Input: part model. Units: mm. Frame: model coordinates. A direction names the side the tool comes from. Round coordinates to 2 decimals unless told otherwise and drop trailing zeros. Order: outer loops, then holes, each group sorted by start corner. A loop starts at its lowest first (then second) coordinate and runs counter-clockwise, first axis right, second up.
Item 1: Mould query, pull axis X, two halves, no side actions, for faces 4 (the flat face through (-10.134, 25, 12)), 5 (the flat face through (5, 28, 25.733)), 6 (the flat face through (17, 19.7, 15)). Classes: released by +X, released by -X, zero draft, split by the parting line, or undercut.
Item 2: Cut plane B-B on x = -0.5. Output: boundary loops of the cut face in (y, z).
Item 3: Reachability of faces 1 (the flat face through (5, 21, 6)), 2 (the flat face through (5.08, 26.44, 26.49)), 3 (the flat face through (5, 28, -1.733)) from +Z, -Z, +X, -X, +Y, -Y: full face, straight path, thin tool, end or side. Return the list, or none.
Item 4: First-contact query: pin 1 (1.5 mm diameter, centred on x = 9.5, z = 4.5, fed in from -Y); pin 2 (1 mm diameter, centred on x = 13, z = 3.5, fed in from +Y); pin 3 (3 mm diameter, centred on x = 15, y = 21, fed in from +Z). Flat tips, straight axial feed; report the tip coordinate or a pass-through.
Item 5: Cut plane A-A on z = 9.5. Output: boundary loops of the cut face in (x, y).
Item 6: Cut plane C-C on z = 20.5. Output: boundary loops of the cut face in (x, y).
Item 7: Line query: L1, parallel to Z at x = 6.5, y = 23; L2, parallel to X at y = 21.2, z = 17.3; L3, parallel to Y at x = 1, z = 17. Output: solid intervals per line, ascending.
Autodesk Inventor part; units mm, degrees
ref_plane "Work Plane3" through (-25.1344, 22.2348, 12) normal (0, 0, -1) x (1, 0, 0)
ref_plane "YZ Plane" through (0, 0, 0) normal (1, 0, 0) x (0, 1, 0)
ref_plane "XZ Plane" through (0, 0, 0) normal (0, 1, 0) x (-1, 0, 0)
sketch "Sketch1" plane through (0, 0, 0) normal (0, 0, 1) x (1, 0, 0)
  circle A0 centre (23.8656, 17.2) radius 3
  line L0 (34.8656, 12.9938) -> (34.8656, 22.2)
  line L1 (165.9417, 25.2) -> (-24.8583, 25.2)
  line L2 (34.8656, 25.2) -> (-24.8606, 25.2)
  line L3 (-24.8606, 25.2) -> (-24.8606, 10.2)
  line L4 (-24.8606, 10.2) -> (34.8656, 10.2)
  line L5 (34.8656, 10.2) -> (34.8656, 25.2)
  point P0 (0, 0)
  dimension "d0" = 15
extrude "Extrusion1" add sketch "Sketch1" along normal blind 4
sketch "Sketch2" plane through (0, 0, 4) normal (0, 0, 1) x (1, 0, 0)
  circle A0 centre (23.8656, 17.2) radius 3
  line L0 (17.8656, 17.2) -> (20.8656, 22.3962)
  line L1 (20.8656, 22.3962) -> (26.8656, 22.3962)
  line L2 (26.8656, 22.3962) -> (29.8656, 17.2)
  line L3 (29.8656, 17.2) -> (26.8656, 12.0038)
  line L4 (26.8656, 12.0038) -> (20.8656, 12.0038)
  line L5 (20.8656, 12.0038) -> (17.8656, 17.2)
  circle A1 centre (23.8656, 17.2) radius 3
  line L6 (34.8656, 25.2) -> (-24.8606, 25.2)
  line L7 (-24.8606, 25.2) -> (-24.8606, 10.2)
  line L8 (-24.8606, 10.2) -> (34.8656, 10.2)
  line L9 (34.8656, 10.2) -> (34.8656, 25.2)
  point P0 (0, 0)
extrude "Extrusion2" add sketch "Sketch2" along normal blind 4 contours L9 L8 L7 L6
sketch "Sketch4" plane through (34.8656, 10.2, 8) normal (1, 0, 0) x (0, 0, -1)
  line L0 (8, 0.0155) -> (-4, 0.0155)
  point P0 (8, -10.2)
  dimension "d8" = 12
sketch "Sketch6" plane through (0, 0, 4) normal (0, 0, 1) x (1, 0, 0)
  line L0 (20.8656, 22.3962) -> (17.8656, 17.2)
  line L1 (17.8656, 17.2) -> (20.8656, 12.0038)
  line L2 (20.8656, 12.0038) -> (26.8656, 12.0038)
  line L3 (26.8656, 12.0038) -> (29.8656, 17.2)
  line L4 (29.8656, 17.2) -> (26.8656, 22.3962)
  circle A0 centre (23.8656, 17.2) radius 3
  line L5 (26.8656, 22.3962) -> (20.8656, 22.3962)
  point P0 (0, 0)
extrude "Extrusion4" cut sketch "Sketch6" along normal blind 16
sketch "Sketch7" plane through (0, 0, 4) normal (0, 0, 1) x (1, 0, 0)
  circle A0 centre (23.8656, 17.2) radius 3
  line L0 (17.8656, 17.2) -> (20.8656, 12.0038)
  line L1 (17.8656, 17.2) -> (20.8656, 22.3962)
  line L2 (20.8656, 22.3962) -> (26.8656, 22.3962)
  line L3 (26.8656, 22.3962) -> (29.8656, 17.2)
  line L4 (29.8656, 17.2) -> (26.8656, 12.0038)
  line L5 (26.8656, 12.0038) -> (20.8656, 12.0038)
  line L6 (20.8656, 12.0038) -> (17.8656, 17.2)
  point P0 (0, 0)
extrude "Extrusion5" cut sketch "Sketch7" along normal blind 16
sketch "Sketch8" plane through (34.8656, 10.2, 0) normal (1, 0, 0) x (0, 0, -1)
  line L0 (-41.5, 15) -> (17.4652, 15)
  line L1 (17.4652, 16) -> (17.4652, 15) construction
  line L2 (15.4652, 18) -> (17.4652, 16) construction
  line L3 (14.5, 18) -> (15.4652, 18) construction
  line L4 (14.5, 18) -> (14.5, 63) construction
  arc A0 (14.5, 63) -> (12.5, 65) centre (12.5, 63) ccw construction
  line L5 (12.5, 65) -> (7.5, 65) construction
  line L6 (7.5, 65) -> (10.5, 62) construction
  line L7 (10.5, 62) -> (10.5, 20) construction
  arc A1 (8.5, 18) -> (10.5, 20) centre (8.5, 20) ccw construction
  line L8 (8.5, 18) -> (-32.5, 18) construction
  arc A2 (-34.5, 20) -> (-32.5, 18) centre (-32.5, 20) ccw construction
  line L9 (-34.5, 20) -> (-34.5, 62) construction
  line L10 (-34.5, 62) -> (-31.5, 65) construction
  line L11 (-31.5, 65) -> (-36.5, 65) construction
  arc A3 (-36.5, 65) -> (-38.5, 63) centre (-36.5, 63) ccw construction
  line L12 (-38.5, 63) -> (-38.5, 18) construction
  line L13 (-38.5, 18) -> (-39.5, 18) construction
  line L14 (-39.5, 18) -> (-41.5, 16) construction
  line L15 (-41.5, 16) -> (-41.5, 15) construction
  line L16 (0, 15) -> (17.4652, 15)
  line L17 (17.4652, 15) -> (18.4652, 15)
  line L18 (18.4652, 15) -> (18.4652, 16)
  line L19 (18.4652, 16) -> (15.4652, 19)
  line L20 (21.4652, 15) -> (21.4652, 18)
  line L21 (17.4652, 22) -> (15.4652, 22)
  line L22 (21.4652, 15) -> (21.4652, 12.0348)
  line L23 (21.4652, 12.0348) -> (0, 12.0348)
  line L24 (21.4652, 18) -> (17.4652, 22)
  line L25 (0, 0) -> (0, 15) construction
  line L26 (-32.6881, 12) -> (-32.6881, -32.4)
  line L27 (0, 12.0348) -> (-12, 12.0348)
  line L28 (-12, 15) -> (0, 15)
  arc A4 (-34.5, 20) -> (-32.5, 18) centre (-32.5, 20) ccw construction
  line L29 (-24, 15) -> (-41.4652, 15)
  line L30 (-41.4652, 15) -> (-42.4652, 15)
  line L31 (-42.4652, 15) -> (-42.4652, 16)
  line L32 (-42.4652, 16) -> (-39.4652, 19)
  line L33 (-45.4652, 15) -> (-45.4652, 18)
  line L34 (-41.4652, 22) -> (-39.4652, 22)
  line L35 (-45.4652, 15) -> (-45.4652, 12.0348)
  line L36 (-45.4652, 12.0348) -> (-24, 12.0348)
  line L37 (-45.4652, 18) -> (-41.4652, 22)
  line L38 (-24, 12.0348) -> (-12, 12.0348)
  line L39 (-12, 15) -> (-24, 15)
  line L40 (18.4652, 15) -> (-42.4652, 15)
  line L41 (21.4652, 12.0348) -> (-45.4652, 12.0348)
  line L42 (-45.4652, 12.0348) -> (-45.4652, 18)
  line L43 (-45.4652, 18) -> (-41.4652, 22)
  line L44 (-41.4652, 22) -> (-39.4652, 22)
  line L45 (-39.4652, 19) -> (-42.4652, 16)
  line L46 (-42.4652, 16) -> (-42.4652, 15)
  line L47 (-42.4652, 15) -> (18.4652, 15)
  line L48 (15.4652, 19) -> (15.4652, 22)
  line L49 (-39.4652, 19) -> (-39.4652, 22)
  point P0 (0, -10.2)
  point P1 (21.4652, 22)
  point P2 (-45.4652, 22)
  dimension "d16" = 3
  dimension "d17" = 4
  dimension "d18" = 4
extrude "Extrusion6" add sketch "Sketch8" against normal blind 60
sketch "Sketch9" plane through (34.8656, 22.2348, 8) normal (0, -1, 0) x (1, 0, 0)
  line L0 (0, -8) -> (0, -29.4652)
  line L1 (-60, -29.4652) -> (-60, 37.4652)
  line L2 (0, -8) -> (-60, -8)
  line L3 (-60, -8) -> (-60, 16)
  line L4 (-60, 16) -> (0, 16)
  line L5 (0, 16) -> (0, -8)
  line L6 (-60, 4) -> (0, 4)
  point P0 (-34.8656, -8)
  dimension "d21" = 24
ref_plane "Work Plane3" through (-25.1344, 22.2348, 12) normal (0, 0, -1) x (1, 0, 0)
mirror "Mirror2" about plane through (-25.1344, 22.2348, 12) normal (0, 0, -1) of "Extrusion1", "Extrusion2"
sketch "Sketch11" plane through (26.9587, 22.2348, 20) normal (0, 0, -1) x (-1, 0, 0)
  circle A0 centre (3.0931, -5.0348) radius 3
  circle A1 centre (3.0931, -5.0348) radius 7
  circle A2 centre (3.0931, -5.0348) radius 3
  line L0 (-3.9069, -5.0348) -> (-0.4069, 1.0273)
  line L1 (-0.4069, 1.0273) -> (6.5931, 1.0273)
  line L2 (6.5931, 1.0273) -> (10.0931, -5.0348)
  line L3 (10.0931, -5.0348) -> (6.5931, -11.097)
  line L4 (6.5931, -11.097) -> (-0.4069, -11.097)
  line L5 (-0.4069, -11.097) -> (-3.9069, -5.0348)
  point P0 (26.9587, -22.2348)
  dimension "d25" = 14
extrude "Extrusion8" cut sketch "Sketch11" along normal blind 16 contours L3 L4 L5 L0 L1 L2
scale "Scale1" factors (0.5, 0.5, 0.5) then translate (2.4328, 12.6, 6) bodies 1
properties part number "TopToBatteryJoint"
From the geometry:
1. face 4: released by -X
1. face 5: zero draft
1. face 6: undercut
2. outline: (17.7, 6) - (23.72, 6) - (23.72, -4.73) - (26.7, -4.73) - (28.7, -2.73) - (28.7, -1.73) - (27.2, -1.73) - (25.7, -3.23) - (25.2, -3.23) - (25.2, 27.23) - (25.7, 27.23) - (27.2, 25.73) - (28.7, 25.73) - (28.7, 26.73) - (26.7, 28.73) - (23.72, 28.73) - (23.72, 18) - (17.7, 18) - (17.7, 14) - (23.72, 14) - (23.72, 10) - (17.7, 10) - close
3. face 1: -Z, +X, -X, -Y
3. face 2: +X, -X
3. face 3: +X, -X, +Y
4. pin 1: stops at y = 23.72
4. pin 2: stops at y = 25.2
4. pin 3: stops at z = 18
5. outline: (-10.13, 23.72) - (-10, 23.72) - (-10, 17.7) - (19.87, 17.7) - (19.87, 25.2) - (-10.13, 25.2) - close; hole (10.87, 21.2) - (12.62, 18.17) - (16.12, 18.17) - (17.87, 21.2) - (16.12, 24.23) - (12.62, 24.23) - close
6. outline: (-10.13, 23.72) - (19.87, 23.72) - (19.87, 25.2) - (-10.13, 25.2) - close
7. L1: z = 6 to 10, 14 to 18
7. L2: x = -10 to 12.87, 15.87 to 19.87
7. L3: y = 17.7 to 25.2
